from build123d import *

# Parameters (mm, degrees)
F0_R          = 11.1125
F1_DEPTH      = 190.5
F2_SIZE       = 3.175
F3_R          = 4.7625
F4_DEPTH      = 25.4
F4_DEPTH_BACK = 25.4
F5_R          = 3.175
F6_DEPTH      = 12.7


with BuildPart() as f1:
    # F0 (on Top) → F1 (new body)
    with BuildSketch(Plane.XY):
        with Locations((-1.1552e-06, 0.1656521781)):
            Circle(F0_R)
    extrude(amount=F1_DEPTH)

    # F2
    f2_edges = [f1.edges().sort_by_distance(p)[0] for p in [
        (-11.112501, 0.165652, 0),
    ]]
    chamfer(f2_edges, length=F2_SIZE)

    # F3 (on Front) → F4 (cut, two sides)
    with BuildSketch(Plane.XZ) as f4_sk:
        with Locations((0, 171.45)):
            Circle(F3_R)
    extrude(amount=-F4_DEPTH, mode=Mode.SUBTRACT)
    extrude(f4_sk.sketch, amount=F4_DEPTH_BACK, mode=Mode.SUBTRACT)

    # F5 (on face) → F6 (cut)
    with BuildSketch(Plane.XY.offset(190.5)):
        Circle(F5_R)
    extrude(amount=-F6_DEPTH, mode=Mode.SUBTRACT)


solid = f1.part
For this review, take the finished solid that the model builds, in its own axes (mm). A direction names the side the tool comes from. Give positions to 0.01 mm unless a question says otherwise; leave off trailing zeros. Loops run counter-clockwise (first coordinate to the right, second up) from the corner with the lowest first, then second, coordinate; pieces in that order, holes last. Notation, with made-up numbers: (69, 83) -> (87, 83) arc R32 cw to (87, 122) -> close; hole circle Ø2 at (59.5, 42). An arc over 180 degrees is marked (long way). One line per question, with ' | ' between items.
1) The part is to be moulded in two halves that separate along Y. For faces 3 (the flat face through (0, 0, 0)), 4 (the cylindrical face through (10.6, 3.5, 95.5)), 5 (the cylindrical face through (-0.69, -3.1, 184.24)), say which applies: +Y half, -Y half, draft (parallel to the pull), parting line (faces both ways), or undercut.
Resolved:
face 3: draft | face 4: parting line | face 5: undercut
2) We need section B-B (z = 146). Write out the cut boundary in (x, y) (1 decimal), plus the area to 3 significant figures.
Resolved:
outline: circle Ø22.2 at (0, 0.2) | area: 388 mm2
3) For faces 1 (the conical face through (7.718, 2.596, 0.154)), 2 (the flat face through (0, 0, 177.8)), list the 3-axis set-ups (+Z, -Z, +X, -X, +Y, -Y) from which the entire face can be reached by the end or side of a thin tool; tool diameter is ignored.
Resolved:
face 1: -Z | face 2: +Z
4) To check wall thickness, follow probe 1 along Z at (x, y) = (0, 6); probe 2 along Y at (x, z) = (0, 184.75) (3 decimals); probe 3 along Z at (x, y) = (4.25, 5.25). State the ranges of each line that lie inside material, in increasing order.
Resolved:
probe 1: z = 0 to 166.69, 176.21 to 190.5 | probe 2: y = -10.947 to -3.175, 3.175 to 11.278 | probe 3: z = 0 to 169.3, 173.6 to 190.5
5) Insertion check: pin 1 Ø7.5 at (x, z) = (0, 171.45) entering from -Y; pin 2 Ø2 at (y, z) = (-1, 105.5) entering from -X; pin 3 Ø2 at (x, z) = (-8.5, 131.5) entering from +Y; pin 4 Ø1 at (x, z) = (1.5, 32) entering from -Y. Each pin has a flat end and moves straight along its axis. Give the tip position at first contact, or say it passes through.
Resolved:
pin 1: passes through | pin 2: stops at x = -11.11 | pin 3: stops at y = 8.37 | pin 4: stops at y = -10.9
6) We need section A-A (z = 171.45). Write out the cut boundary in (x, y) (1 decimal), plus the area to 3 significant figures.
Resolved:
outline: (-4.8, -9.9) -> (-4.8, 10.2) arc R11.1 ccw to start; (4.8, -9.9) arc R11.1 ccw to (4.8, 10.2) -> close | area: 183 mm2
